Design review of the part shown in the three views and the two pictorial views. Dimensions are in mm from the part's minimum x, y and z. A direction names the side the tool comes from. Round coordinates to 2 decimals unless told otherwise and drop trailing zeros. Loops run counter-clockwise (first coordinate to the right, second up) from the corner with the lowest first, then second, coordinate; pieces in that order, holes last. Notation, with made-up numbers: M 29.5,-24 L 57.5,-24 A19 ccw 57.5,-10 Z; hole C 82.5,40.25 d3. An arc over 180 degrees is marked long. Return JSON: item names as keys, results as strings. Group by question number.
Q1. Consider section A-A (x = 8). State the section outline as (y, z) points (1 decimal).
Q2. Consider section B-B (x = 7). State the section outline as (y, z) points.
Q3. Clearance check with flat-ended pins moving along their axes: pin 1 Ø4 at (y, z) = (1, 1.5) entering from -X; pin 2 Ø2 at (x, z) = (3.5, 2) entering from +Y (1 decimal); pin 3 Ø2 at (y, z) = (4, 3) entering from +X (1 decimal). State where each tip first meets the part, or that it passes through.
Q4. Consider section C-C (x = 5.25). State the section outline as (y, z) points (1 decimal).
Q5. To check wall thickness, follow line 1 along Y through (x, z) = (9.25, 3.5) (1 decimal); line 2 along Z through (x, y) = (7.5, 2.5) (1 decimal); line 3 along X through (y, z) = (1.75, 3.5). State the ranges of each line that lie inside material, in increasing order.
Q6. For the marked faces 1, 2 and 3, list the 3-axis set-ups (+Z, -Z, +X, -X, +Y, -Y) from which the entire face can be reached by the end or side of a thin tool; tool diameter is ignored.
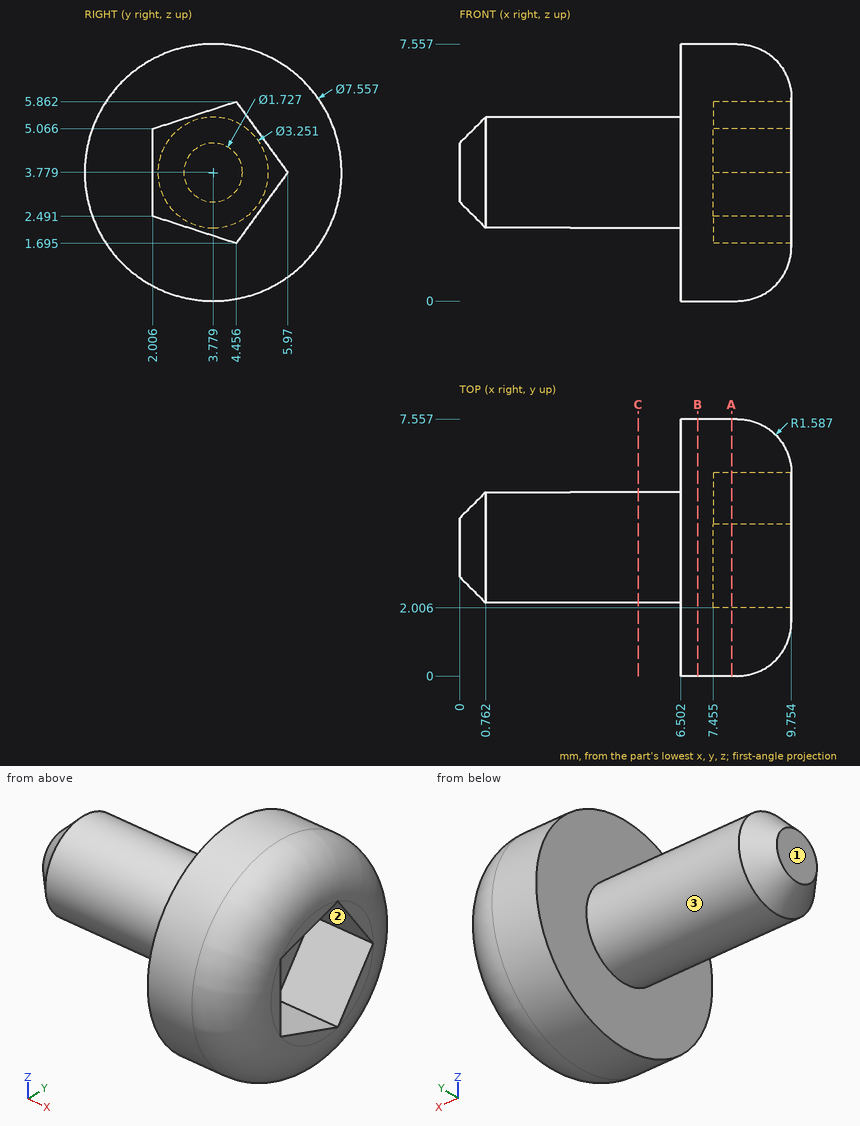
Values:
{
 "1": {"outline": "C 3.8,3.8 d7.6; hole M 2,2.5 L 4.5,1.7 L 6,3.8 L 4.5,5.9 L 2,5.1 Z"},
 "2": {"outline": "C 3.78,3.78 d7.56"},
 "3": {"pin 1": "stops at x = 0.73", "pin 2": "stops at y = 5.2", "pin 3": "stops at x = 7.5"},
 "4": {"outline": "C 3.8,3.8 d3.3"},
 "5": {"line 1": "y = 0.4 to 2, 5.8 to 7.1", "line 2": "z = 0.2 to 2.3, 5.2 to 7.3", "line 3": "x = 6.5 to 9.75"},
 "6": {"face 1": "+Z, -Z, -X, +Y, -Y", "face 2": "+X", "face 3": "-X"}
}
